Answer from the drawing. Dimensions are ordinates in mm from the lowest x, y and z of the part. Round coordinates to 2 decimals unless told otherwise and drop trailing zeros. Order: outer loops, then holes, each group sorted by start corner. A loop starts at its lowest first (then second) coordinate and runs counter-clockwise, first axis right, second up. Notation, with made-up numbers: M 23.5,42 L 64.5,42 A6 cw 64.5,51 Z; hole C 55,19.25 d8. An arc over 180 degrees is marked long. Write item = value, one per line. Start each with the question number.
(1) A cutting plane is placed at B-B, the plane z = 27. Determine the outline of the cut face in (x, y).
(2) A cutting plane is placed at C-C, the plane z = 23. Determine the outline of the cut face in (x, y), and give its area (3 significant figures).
(3) A cutting plane is placed at A-A, the plane x = 6.5. Determine the outline of the cut face in (y, z).
(4) Straight lines are drawn through the part: probe 1 along Y at (x, z) = (27, 27); probe 2 along Y at (x, z) = (22.25, 22.5). For each, find the intervals that lie inside material, in ascending order. Write a range as from..to.
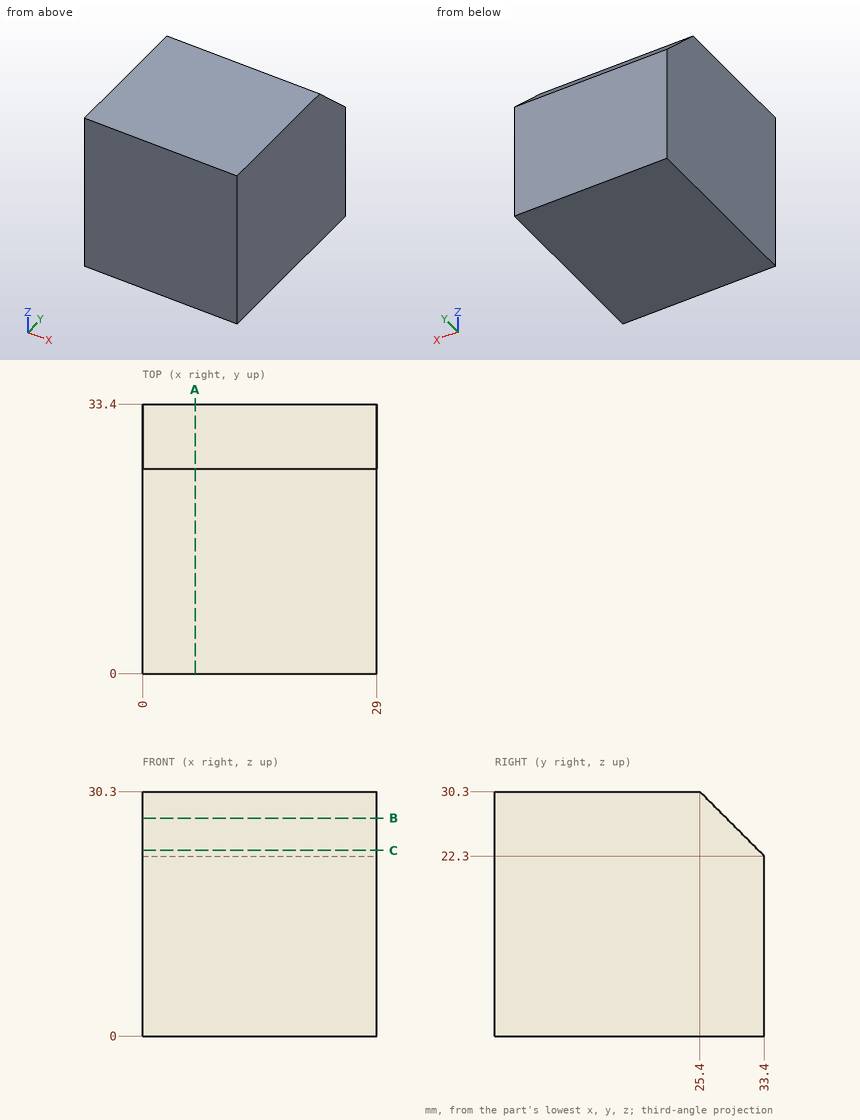
Reported:
q1.outline = M 0,0 L 29,0 L 29,28.7 L 0,28.7 Z
q2.outline = M 0,0 L 29,0 L 29,32.7 L 0,32.7 Z
q2.area = 948 mm²
q3.outline = M 0,0 L 33.4,0 L 33.4,22.3 L 25.4,30.3 L 0,30.3 Z
q4.probe_1 = 0..28.7
q4.probe_2 = 0..33.2
